from build123d import *

# Parameters (mm, degrees)
ESQUISSE1_R        = 1.101038198
ESQUISSE1_R_2      = 0.6
ESQUISSE1_R_3      = 0.753706931
ESQUISSE1_R_4      = 0.470708968
BOSS_EXTRU_1_DEPTH = 0.5


with BuildPart() as part:
    # Esquisse1 → Boss.-Extru.1 (new body)
    with BuildSketch(Plane.XY):
        with BuildLine():
            Line((4.327755202, 9.268221518), (3.603132185, 4.253126908))
            add(Edge.make_bspline(
                [(3.603132185, 4.253126908), (3.97023948, 3.660792989), (4.479491264, 3.174109207), (5.130887536, 2.793075563)],
                knots=[0.419081869, 0.419081869, 0.419081869, 0.419081869, 1, 1, 1, 1], degree=3))
            add(Edge.make_bspline(
                [(5.130887536, 2.793075563), (7.24661574, -1.876356548), (6.801291284, -6.882931027)],
                knots=[0, 0, 0, 1, 1, 1], degree=2))
            Line((6.801291284, -6.882931027), (8.047479128, -3.441465514))
            add(Edge.make_bspline(
                [(7.993289874, 10.651808238), (10.006516758, 3.73495856), (8.047479128, -3.441465514)],
                knots=[0, 0, 0, 1, 1, 1], degree=2))
            add(Edge.make_bspline(
                [(7.993289874, 10.651808238), (7.437530526, 13.742255062), (4.969978084, 15.276811926)],
                knots=[0, 0, 0, 1, 1, 1], degree=2))
            add(Edge.make_bspline(
                [(4.969978084, 15.276811926), (6.336855169, 14.093829897), (6.151102735, 12.493995378)],
                knots=[0, 0, 0, 1, 1, 1], degree=2))
            add(Edge.make_bspline(
                [(6.151102735, 12.493995378), (5.8933943, 11.152214383), (5.285611789, 10.07695643), (4.327755202, 9.268221518)],
                knots=[0, 0, 0, 0, 0.717084893, 0.717084893, 0.717084893, 0.717084893], degree=3))
        make_face()
        with Locations((7.16473136, 3.33945502)):
            Circle(ESQUISSE1_R, mode=Mode.SUBTRACT)
        with Locations((5.43038475, 8.539470271)):
            Circle(ESQUISSE1_R_2, mode=Mode.SUBTRACT)
        with Locations((7.47952091, 0.328032682)):
            Circle(ESQUISSE1_R_3, mode=Mode.SUBTRACT)
        with Locations((7.586653272, -2.053387377)):
            Circle(ESQUISSE1_R_4, mode=Mode.SUBTRACT)
        with Locations((4.969978084, 4.416971754)):
            Circle(ESQUISSE1_R_2, mode=Mode.SUBTRACT)
    extrude(amount=BOSS_EXTRU_1_DEPTH)


solid = part.part
Design review of the part built by this model. Coordinates are the model's own, in mm. Round coordinates to 2 decimals unless told otherwise and drop trailing zeros. One line per item, written item: value. Start each with the question number.
1) Insertion check: pin 1 Ø1.6 at (x, y) = (4.97, 4.42) entering from +Z. The pin has a flat end and moves straight along its axis. Give the tip position at first contact, or say it passes through.
2) To check wall thickness, follow L1, parallel to X at y = 9, z = 0.15; L2, parallel to X at y = 5.75, z = 0.4; L3, parallel to X at y = -5, z = 0.2. State the ranges of each line that lie inside material, in increasing order. Write a range as from..to.
3) Draft analysis for pull direction Y (two halves, no side actions). For faces 1 (the cylindrical face through (6.727, 0.361, 0.246)), 2 (the flat face through (7.416, -5.186, 0.246)), 3 (the flat face through (7, 7, 0)), state which applies: +Y half, -Y half, draft (parallel to the pull), parting line (faces both ways), or undercut.
4) Consider section A-A on x = 7.6. Give the number of separate pieces and of enclosed holes in the cut face, then the cut area to 3 significant figures.
Reported:
1. pin 1: stops at z = 0.5
2. L1: x = 4.29..5.05, 5.81..8.42
2. L2: x = 3.82..8.92
2. L3: x = 6.88..7.48
3. face 1: undercut
3. face 2: -Y half
3. face 3: draft
4. separate pieces: 4
4. enclosed holes: 0
4. area: 6.16 mm^2
